from build123d import *

# Parameters (mm, degrees)
F1_DEPTH  = 20
F2_R      = 4.25
F2_R_2    = 1.395
F3_DEPTH  = 30
F2_R_3    = 5.5
F4_DEPTH  = 2
F6_DEPTH  = 25
F8_DEPTH  = 10.001
F10_DEPTH = 15


with BuildPart() as f1:
    # F0 (on Front) → F1 (new body)
    with BuildSketch(Plane.XZ):
        with BuildLine():
            Line((29.9143858576, 52.0108596234), (0, 0))
            Line((0, 0), (130, 0))
            Line((130, 0), (130, 10))
            Line((130, 10), (88.2409628552, 10))
            ThreePointArc((88.2409628552, 10), (83.0804911789, 10.6772276296), (78.2695009027, 12.6630467922))
            Line((78.2695009027, 12.6630467922), (62.2031042781, 21.9037398215))
            ThreePointArc((62.2031042781, 21.9037398215), (61.5027165088, 22.8133971511), (61.650692434, 23.9518709585))
            Line((61.650692434, 23.9518709585), (62.1492655316, 24.8187186189))
            Line((62.1492655316, 24.8187186189), (44.8123123238, 34.7901805715))
            Line((44.8123123238, 34.7901805715), (44.3137392262, 33.9233329111))
            ThreePointArc((44.3137392262, 33.9233329111), (43.4040818966, 33.2229451418), (42.2656080891, 33.3709210669))
            Line((42.2656080891, 33.3709210669), (27.5291978625, 41.8466637266))
            ThreePointArc((27.5291978625, 41.8466637266), (26.8288100932, 42.7563210562), (26.9767860184, 43.8947948636))
            Line((26.9767860184, 43.8947948636), (31.2146573482, 51.2629999769))
            Line((31.2146573482, 51.2629999769), (29.9143858576, 52.0108596234))
        make_face()
        with BuildLine():
            Line((27.7705867405, 1.3316440692), (13.1131062569, 9.7619897713))
            ThreePointArc((13.1131062569, 9.7619897713), (10.7784803592, 12.7941808699), (11.2717334431, 16.5890935613))
            Line((11.2717334431, 16.5890935613), (22.9882012374, 36.9600135805))
            ThreePointArc((22.9882012374, 36.9600135805), (26.020392336, 39.2946394782), (29.8153050274, 38.8013863943))
            Line((29.8153050274, 38.8013863943), (78.5948983283, 10.7454844818))
            ThreePointArc((78.5948983283, 10.7454844818), (80.9337866185, 5.1251064419), (76.1102671502, 1.4112529602))
            Line((76.1102671502, 1.4112529602), (27.7705867405, 1.3316440692))
        make_face(mode=Mode.SUBTRACT)
    extrude(amount=F1_DEPTH)

    # F2 (on face) → F3 (cut)
    with BuildSketch(Plane(origin=(0, 0, 0), x_dir=(0, -1, 0), z_dir=(-0.8668476604, 0, 0.4985730976))):
        with Locations((10, 7.5)):
            Circle(F2_R)
        with Locations((5, 39)):
            Circle(F2_R_2)
        with Locations((5, 32)):
            Circle(F2_R_2)
        with Locations((15, 32)):
            Circle(F2_R_2)
        with Locations((15, 39)):
            Circle(F2_R_2)
        with Locations((5, 25)):
            Circle(F2_R_2)
        with Locations((15, 25)):
            Circle(F2_R_2)
    extrude(amount=-F3_DEPTH, mode=Mode.SUBTRACT)

    # F2 (on face) → F4 (cut)
    with BuildSketch(Plane(origin=(0, 0, 0), x_dir=(0, -1, 0), z_dir=(-0.8668476604, 0, 0.4985730976))):
        with Locations((10, 7.5)):
            Circle(F2_R_3)
        with Locations((10, 7.5)):
            Circle(F2_R, mode=Mode.SUBTRACT)
    extrude(amount=-F4_DEPTH, mode=Mode.SUBTRACT)

    # F5 (on face) → F6 (cut)
    with BuildSketch(Plane.XY.offset(10)):
        with BuildLine():
            Line((95, -18), (95, -20))
            Line((95, -20), (130, -20))
            Line((130, -20), (130, -15))
            Line((130, -15), (98, -15))
            ThreePointArc((98, -15), (95.8786796564, -15.8786796564), (95, -18))
        make_face()
        with BuildLine():
            Line((130, 0), (95, 0))
            Line((95, 0), (95, -2))
            ThreePointArc((95, -2), (95.8786796564, -4.1213203436), (98, -5))
            Line((98, -5), (130, -5))
            Line((130, -5), (130, 0))
        make_face()
    extrude(amount=-F6_DEPTH, mode=Mode.SUBTRACT)

    # F7 (on face) → F8 (cut, through all)
    with BuildSketch(Plane.XY.offset(10)):
        with BuildLine():
            Line((130, -13), (130, -7))
            Line((130, -7), (113, -7))
            ThreePointArc((113, -7), (110, -10), (113, -13))
            Line((113, -13), (130, -13))
        make_face()
    extrude(amount=-F8_DEPTH, mode=Mode.SUBTRACT)

    # F9 (on face) → F10 (cut)
    with BuildSketch(Plane(origin=(26.1750876254, 0, 45.5095021704), x_dir=(0.8668476604, 0, -0.4985730976), z_dir=(0.4985730976, 0, 0.8668476604))):
        with BuildLine():
            ThreePointArc((28, -6), (24, -10), (28, -14))
            Line((28, -14), (35, -14))
            ThreePointArc((35, -14), (39, -10), (35, -6))
            Line((35, -6), (28, -6))
        make_face()
    extrude(amount=-F10_DEPTH, mode=Mode.SUBTRACT)


solid = f1.part
Input: part model. Units: mm. Frame: model coordinates. A direction names the side the tool comes from. Coordinates: 2 decimals unless noted, no trailing zeros. Loops run counter-clockwise (first coordinate to the right, second up) from the corner with the lowest first, then second, coordinate; pieces in that order, holes last. Notation, with made-up numbers: (1.5, -26.75) -> (11.5, -26.75) arc R32 cw to (11.5, 12.25) -> close; hole circle Ø9 at (-20, 84). An arc over 180 degrees is marked (long way). One line per item, written item: value.
(1) Pin query (flat end, axial travel): pin 1 Ø2 at (y, z) = (-1, 3) entering from +X; pin 2 Ø7.5 at (x, z) = (53.5, 26.5) entering from +Y; pin 3 Ø6 at (x, y) = (106.5, -9) entering from +Z; pin 4 Ø5 at (x, z) = (114, 4.5) entering from -Y. Return the tip coordinate at first contact, or that it passes through.
Answer below:
pin 1: stops at x = 95
pin 2: stops at y = 0
pin 3: stops at z = 10
pin 4: stops at y = -15
(2) Cut plane C-C (x = 107.5). Output: boundary loops of the cut face in (y, z), then the cut area to 3 significant figures.
Answer below:
outline: (-15, 0) -> (-5, 0) -> (-5, 10) -> (-15, 10) -> close
area: 100 mm2
(3) Ray query, line 1 along Z through (x, y) = (28.5, -0.75); line 2 along X through (y, z) = (-2, 13.5); line 3 along X through (y, z) = (-10.75, 5). Return the intervals inside material, ascending.
Answer below:
line 1: z = 0 to 1.33, 39.33 to 41.29, 46.54 to 49.55
line 2: x = 7.76 to 10.64, 73.81 to 76.81
line 3: x = 14.74 to 21.39, 80.9 to 110.1
(4) Cut plane D-D (z = 49). Output: boundary loops of the cut face in (x, y).
Answer below:
outline: (28.18, -20) -> (29.91, -20) -> (29.91, 0) -> (28.18, 0) -> close
(5) Set-up query: faces 1 (the face through (45.997, -9.912, 31.834)), 2 (the face through (80.957, -9.86, 5.214)), 3 (the face through (13.67, -9.45, 5.65)), 4 (the face through (105, -10, 10)), 5 (the face through (44, 0, 1)). Return all of +Z, -Z, +X, -X, +Y, -Y with unobstructed straight access to the full face (end or side cutting, diameter ignored); none if empty.
Answer below:
face 1: +X
face 2: +Y, -Y
face 3: none
face 4: +Z, +X, +Y, -Y
face 5: +Z, -Z, +X, -X, +Y
(6) Cut plane A-A (x = 41). Output: boundary loops of the cut face in (y, z), then the cut area to 3 significant figures.
Answer below:
outline: (-20, 0) -> (0, 0) -> (0, 1.35) -> (-20, 1.35) -> close; (-20, 32.37) -> (0, 32.37) -> (0, 34.1) -> (-20, 34.1) -> close
area: 61.7 mm2
(7) Draft query along X for faces 6 (the face through (17.048, -9.86, 26.632)), 7 (the face through (110, -10, 5)), 8 (the face through (20.54, -9.86, 5.49)), 9 (the face through (114, -5, 5)). Return one class per face: pulls with the +X half, pulls with the -X half, needs draft (parallel to the pull), parting line crosses it, or undercut.
Answer below:
face 6: undercut
face 7: pulls with the +X half
face 8: undercut
face 9: needs draft
